from build123d import *

# Parameters (mm, degrees)
F1_DEPTH = 5
F2_R     = 7.46933
F3_DEPTH = 25


with BuildPart() as f1:
    # F0 (on Front) → F1 (new body)
    with BuildSketch(Plane.XZ):
        Polygon((9.318711, 3.08139), (1.990793, 9.610935), (-7.327917, 6.529545), (-9.318711, -3.08139), (-1.990793, -9.610935), (7.327917, -6.529545), align=None)
    extrude(amount=F1_DEPTH)

    # F2 (on face) → F3 (join)
    with BuildSketch(Plane(origin=(0, 0, 0), x_dir=(-1, 0, 0), z_dir=(0, 1, 0))):
        Circle(F2_R)
    extrude(amount=F3_DEPTH)


solid = f1.part
Check sheet for the modelled part. Datum: model origin and axes. Units: mm. A direction names the side the tool comes from. Give positions to 0.01 mm unless a question says otherwise; leave off trailing zeros. Write each loop counter-clockwise with the first axis right and the second up, starting at its lowest first coordinate (ties: lowest second). Pieces come first, ordered by that corner, then holes. Notation, with made-up numbers: (88.25, 10) -> (119.25, 10) arc R11 cw to (119.25, 14) -> close; hole circle Ø5 at (16, 50.25). An arc over 180 degrees is marked (long way). Write item = value, one per line.
Item 1: Gauge pin test, flat end, axial feed: pin 1 (4 mm diameter, centred on y = 5, z = 3, fed in from -X). Record the tip position at first contact, or that the pin passes through.
Output:
pin_1 = -7.4
Item 2: Sectioned sample at C-C on x = -0.5. Record the boundary of the cut face in (y, z), and give its area (3 significant figures).
Output:
outline = (-5, -9.12) -> (0, -9.12) -> (0, -7.45) -> (25, -7.45) -> (25, 7.45) -> (0, 7.45) -> (0, 8.79) -> (-5, 8.79) -> close
area = 462 mm^2
Item 3: Sectioned sample at D-D on y = 5.25. Record the boundary of the cut face in (x, z), and give its area (3 significant figures).
Output:
outline = circle Ø14.94 at (0, 0)
area = 175 mm^2
Item 4: Scan lines: probe 1 along X at (y, z) = (19, 0.25); probe 2 along Y at (x, z) = (7.75, 4.25); probe 3 along X at (y, z) = (13, 1). Record each from-to range of solid material in increasing order. Write a range as from..to.
Output:
probe_1 = -7.47..7.47
probe_2 = -5..0
probe_3 = -7.4..7.4
Item 5: Sectioned sample at A-A on y = -3. Record the boundary of the cut face in (x, z).
Output:
outline = (-9.32, -3.08) -> (-1.99, -9.61) -> (7.33, -6.53) -> (9.32, 3.08) -> (1.99, 9.61) -> (-7.33, 6.53) -> close
Item 6: Sectioned sample at B-B on z = 5.25. Record the boundary of the cut face in (x, y), and give its area (3 significant figures).
Output:
outline = (-7.59, -5) -> (6.88, -5) -> (6.88, 0) -> (5.31, 0) -> (5.31, 25) -> (-5.31, 25) -> (-5.31, 0) -> (-7.59, 0) -> close
area = 338 mm^2
Item 7: Tool access check on faces 1 (the cylindrical face through (-4.015, 12.325, 6.298)), 2 (the flat face through (0, 25, 0)). Record the directions out of +Z, -Z, +X, -X, +Y, -Y that give a thin tool (end or side, any length) a straight path to the whole face; none if there is none.
Output:
face_1 = +Y
face_2 = +Z, -Z, +X, -X, +Y
